```python
from build123d import *

# Parameters (mm, degrees)
F0_R     = 1.5
F0_R_2   = 2.334565
F1_DEPTH = 3


with BuildPart() as f1:
    # F0 (on Top) → F1 (new body)
    with BuildSketch(Plane.XY):
        with BuildLine():
            ThreePointArc((-65, 0), (-62.949747, -4.949747), (-58, -7))
            Line((-58, -7), (58, -7))
            ThreePointArc((58, -7), (62.949747, -4.949747), (65, 0))
            ThreePointArc((65, 0), (62.949747, 4.949747), (58, 7))
            Line((58, 7), (-58, 7))
            ThreePointArc((-58, 7), (-62.949747, 4.949747), (-65, 0))
        make_face()
        with Locations((-58, 0)):
            Circle(F0_R, mode=Mode.SUBTRACT)
        with Locations((-28, 0)):
            Circle(F0_R, mode=Mode.SUBTRACT)
        with Locations((58, 0)):
            Circle(F0_R_2, mode=Mode.SUBTRACT)
    extrude(amount=F1_DEPTH)


solid = f1.part
```
The listing builds one solid part. Answer for the finished solid, in the listing's coordinates (mm). Coordinates: 2 decimals unless noted, no trailing zeros. Write each loop counter-clockwise with the first axis right and the second up, starting at its lowest first coordinate (ties: lowest second). Pieces come first, ordered by that corner, then holes. Notation, with made-up numbers: M -26,52.25 L 9,52.25 A34 cw 9,88.25 Z; hole C -25.5,70 d5. An arc over 180 degrees is marked long. Use a Markdown table: item, result. Add a question column.
1. Section D-D (y = -5.75) is taken. Give the vertices of the cut face in (x, z), plus the area to 3 significant figures.
2. Straight lines are drawn through the part: line 1 along Y through (x, z) = (-28, 2.2); line 2 along Y through (x, z) = (58, 0.9); line 3 along X through (y, z) = (0.75, 2.45). For each, find the intervals that lie inside material, in ascending order. Write a range as [from, to].
3. Section B-B (x = -28) is taken. Give the vertices of the cut face in (y, z).
4. Section C-C (y = 4.5) is taken. Give the vertices of the cut face in (x, z).
5. For a pull along Y with two mould halves and no side action, classify faces 1 (the cylindrical face through (-29.5, 0.07, 1.48)), 2 (the flat face through (-1, -7, 1)), 3 (the flat face through (1, 7, 1)), 4 (the flat face through (-1, 0, 3)) as +Y half, -Y half, draft (parallel to the pull), parting line (faces both ways), or undercut.
6. Section A-A (z = 0.9) is taken. Give the vertices of the cut face in (x, y), plus the area to 3 significant figures.
Data:
| question | item | result |
|---|---|---|
| 1 | outline | M -61.99,0 L 61.99,0 L 61.99,3 L -61.99,3 Z |
| 1 | area | 372 mm2 |
| 2 | line 1 | y = [-7, -1.5], [1.5, 7] |
| 2 | line 2 | y = [-7, -2.33], [2.33, 7] |
| 2 | line 3 | x = [-64.96, -59.3], [-56.7, -29.3], [-26.7, 55.79], [60.21, 64.96] |
| 3 | outline | M -7,0 L -1.5,0 L -1.5,3 L -7,3 Z; M 1.5,0 L 7,0 L 7,3 L 1.5,3 Z |
| 4 | outline | M -63.36,0 L 63.36,0 L 63.36,3 L -63.36,3 Z |
| 5 | face 1 | undercut |
| 5 | face 2 | -Y half |
| 5 | face 3 | +Y half |
| 5 | face 4 | draft |
| 6 | outline | M -65,0 A7 ccw -58,-7 L 58,-7 A7 ccw 65,0 A7 ccw 58,7 L -58,7 A7 ccw Z; hole C -58,0 d3; hole C -28,0 d3; hole C 58,0 d4.67 |
| 6 | area | 1,750 mm2 |
